Input: part model. Units: mm. Frame: model coordinates. A direction names the side the tool comes from. Coordinates: 2 decimals unless noted, no trailing zeros. Write each loop counter-clockwise with the first axis right and the second up, starting at its lowest first coordinate (ties: lowest second). Pieces come first, ordered by that corner, then holes. Notation, with made-up numbers: (-33.5, 74) - (-5.5, 74) arc R25 ccw to (-5.5, 89) - close; hole circle Ø10 at (83.5, 69.25). An arc over 180 degrees is marked (long way). Put each result on its own line as item: value. Start each with the question number.
1. Line query: line 1 (X direction, y = -51, z = 0.4); line 2 (X direction, y = 87.5, z = 1.5) (3 decimals); line 3 (Y direction, x = 9.25, z = 0.55). Output: solid intervals per line, ascending.
2. Cut plane A-A, the plane y = -48. Return loops of the section in (x, z), and give its area (3 significant figures).
3. Access query for faces 1 (the flat face through (-2.4, 1.5, 0)), 2 (the cylindrical face through (0.1, 83.5, 1)). Directions: +Z, -Z, +X, -X, +Y, -Y. A direction counts if a zero-diameter tool reaches every point of the face in a straight line with its end or side. Return the directions, or none.
4. Cut plane B-B, the plane z = 0.7. Count the separate pieces of the cut face and the enclosed holes in it, and give its area (3 significant figures).
5. Pull-direction query (Y, two-part tool) for faces 3 (the flat face through (-2.4, 1.5, 2)), 4 (the cylindrical face through (-0.59, 102.96, 1.01)); classes: released by +Y, released by -Y, zero draft, split by the parting line, or undercut.
from build123d import *

# Parameters (mm, degrees)
SKETCH_1_W          = 20
SKETCH_1_H          = 215
EXTRUDE_1_DEPTH     = 2
FILLET_1_R          = 2
SKETCH_2_R          = 1.525
CUT_EXTRUDE_1_DEPTH = 10
SKETCH_4_R          = 4.5
CUT_EXTRUDE_2_DEPTH = 10


with BuildPart() as part:
    # 草图1 → 凸台-拉伸1 (new body)
    with BuildSketch(Plane.XY):
        Rectangle(SKETCH_1_W, SKETCH_1_H)
    extrude(amount=EXTRUDE_1_DEPTH)

    # 圆角1
    fillet_1_edges = [part.edges().sort_by_distance(p)[0] for p in [
        (10, -107.5, 1),
        (-10, -107.5, 1),
        (-10, 107.5, 1),
        (10, 107.5, 1),
    ]]
    fillet(fillet_1_edges, radius=FILLET_1_R)

    # 草图2 → 切除-拉伸1 (cut)
    with BuildSketch(Plane.XY.offset(2)):
        with Locations((0, 87.5)):
            Circle(SKETCH_2_R)
        with Locations((0, 57.5)):
            Circle(SKETCH_2_R)
        with Locations((0, 27.5)):
            Circle(SKETCH_2_R)
        with Locations((0, -2.5)):
            Circle(SKETCH_2_R)
        with Locations((0, -32.5)):
            Circle(SKETCH_2_R)
        with Locations((0, -62.5)):
            Circle(SKETCH_2_R)
        with Locations((0, -92.5)):
            Circle(SKETCH_2_R)
    extrude(amount=-CUT_EXTRUDE_1_DEPTH, mode=Mode.SUBTRACT)

    # 草图4 → 切除-拉伸2 (cut)
    with BuildSketch(Plane.XY.offset(2)):
        with Locations((0, 98.5)):
            Circle(SKETCH_4_R)
        with BuildLine():
            Line((5, 66.5), (5, 78.5))
            ThreePointArc((5, 78.5), (0, 83.5), (-5, 78.5))
            Line((-5, 78.5), (-5, 66.5))
            ThreePointArc((-5, 66.5), (0, 61.5), (5, 66.5))
        make_face()
        with BuildLine():
            Line((5, 36.5), (5, 48.5))
            ThreePointArc((5, 48.5), (0, 53.5), (-5, 48.5))
            Line((-5, 48.5), (-5, 36.5))
            ThreePointArc((-5, 36.5), (0, 31.5), (5, 36.5))
        make_face()
        with BuildLine():
            Line((5, -83.5), (5, -71.5))
            ThreePointArc((5, -71.5), (0, -66.5), (-5, -71.5))
            Line((-5, -71.5), (-5, -83.5))
            ThreePointArc((-5, -83.5), (0, -88.5), (5, -83.5))
        make_face()
        with BuildLine():
            Line((5, 6.5), (5, 18.5))
            ThreePointArc((5, 18.5), (0, 23.5), (-5, 18.5))
            Line((-5, 18.5), (-5, 6.5))
            ThreePointArc((-5, 6.5), (0, 1.5), (5, 6.5))
        make_face()
        with BuildLine():
            Line((5, -23.5), (5, -11.5))
            ThreePointArc((5, -11.5), (0, -6.5), (-5, -11.5))
            Line((-5, -11.5), (-5, -23.5))
            ThreePointArc((-5, -23.5), (0, -28.5), (5, -23.5))
        make_face()
        with BuildLine():
            Line((5, -53.5), (5, -41.5))
            ThreePointArc((5, -41.5), (0, -36.5), (-5, -41.5))
            Line((-5, -41.5), (-5, -53.5))
            ThreePointArc((-5, -53.5), (0, -58.5), (5, -53.5))
        make_face()
    extrude(amount=-CUT_EXTRUDE_2_DEPTH, mode=Mode.SUBTRACT)


solid = part.part
Report:
1. line 1: x = -10 to -5, 5 to 10
1. line 2: x = -10 to -1.525, 1.525 to 10
1. line 3: y = -107.06 to 107.06
2. outline: (-10, 0) - (-5, 0) - (-5, 2) - (-10, 2) - close; (5, 0) - (10, 0) - (10, 2) - (5, 2) - close
2. area: 20.0 mm^2
3. face 1: -Z, +X, -X, +Y, -Y
3. face 2: +Z, -Z
4. separate pieces: 1
4. enclosed holes: 14
4. area: 2,990 mm^2
5. face 3: zero draft
5. face 4: undercut
